Read the model definition and answer for the solid it produces. Units are mm, in the model's axes. Face numbers are marked on the shaded views. Give positions to 0.01 mm unless a question says otherwise; leave off trailing zeros. Order: outer loops, then holes, each group sorted by start corner. A loop starts at its lowest first (then second) coordinate and runs counter-clockwise, first axis right, second up. Notation, with made-up numbers: (4.5, 2) -> (27.5, 2) arc R22 ccw to (27.5, 10) -> close; hole circle Ø11 at (11.25, -38). An arc over 180 degrees is marked (long way). One line per question, with ' | ' between items. Start each with the question number.
```python
from build123d import *

# Parameters (mm, degrees)
PAD_DEPTH       = 5
SKETCH001_R     = 2.65
POCKET_DEPTH    = 5
SKETCH002_R     = 1.5
POCKET001_DEPTH = 5


with BuildPart() as part:
    # Sketch → Pad (new body)
    with BuildSketch(Plane.XY):
        Polygon((38.75, 34.75), (38.75, -34.75), (26.25, -34.75), (26.25, -45), (-38.75, -45), (-38.75, 45), (26.25, 45), (26.25, 34.75), align=None)
    extrude(amount=PAD_DEPTH)

    # Sketch001 (on Face10 of Pad) → Pocket (cut)
    with BuildSketch(Plane.XY.offset(5)):
        with Locations((31.25, 20)):
            Circle(SKETCH001_R)
        with Locations((31.25, -20)):
            Circle(SKETCH001_R)
    extrude(amount=-POCKET_DEPTH, mode=Mode.SUBTRACT)

    # Sketch002 (on Face5 of Pocket) → Pocket001 (cut)
    with BuildSketch(Plane.XY.offset(5)):
        with Locations((5.25, -16.5)):
            Circle(SKETCH002_R)
        with Locations((-16.75, -16.5)):
            Circle(SKETCH002_R)
        with Locations((-5.75, 15.5)):
            Circle(SKETCH002_R)
    extrude(amount=-POCKET001_DEPTH, mode=Mode.SUBTRACT)


solid = part.part
```
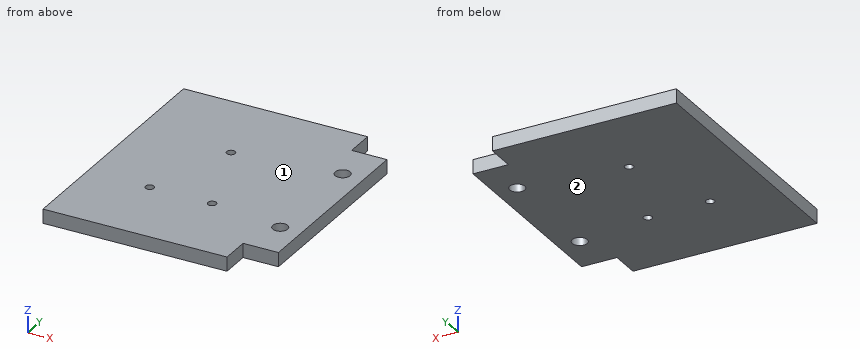
Q1. A cutting plane is placed at B-B, the plane y = -20. Determine the outline of the cut face in (x, z).
Q2. A cutting plane is placed at A-A, the plane x = 31.25. Determine the outline of the cut face in (y, z).
Q3. A cutting plane is placed at D-D, the plane x = 5.25. Determine the outline of the cut face in (y, z).
Q4. A cutting plane is placed at C-C, the plane z = 3.1. Determine the outline of the cut face in (x, y).
Q5. Given P1, Ø1.5, axis at x = 33.5, z = 1.5, coming from the +Y side; P2, Ø2.5, axis at x = 34, z = 1.5, coming from the -Y side; P3, Ø2.5, axis at y = 41.5, z = 2.5, coming from the +X side, each flat-ended and moving along its own axis, determine where each tip first touches the part or whether it passes through.
Q6. Determine the mould class of the marked faces 1 and 2 for opening direction Z: pulls with the +Z half, pulls with the -Z half, needs draft (parallel to the pull), parting line crosses it, or undercut.
Q7. Find the intervals of material crossed by line 1 (Y direction, x = 31.25, z = 3.6); line 2 (Y direction, x = -16.5, z = 2.6); line 3 (Y direction, x = -5.75, z = 1.65), in increasing order.
Geometry results:
1) outline: (-38.75, 0) -> (28.6, 0) -> (28.6, 5) -> (-38.75, 5) -> close; (33.9, 0) -> (38.75, 0) -> (38.75, 5) -> (33.9, 5) -> close
2) outline: (-34.75, 0) -> (-22.65, 0) -> (-22.65, 5) -> (-34.75, 5) -> close; (-17.35, 0) -> (17.35, 0) -> (17.35, 5) -> (-17.35, 5) -> close; (22.65, 0) -> (34.75, 0) -> (34.75, 5) -> (22.65, 5) -> close
3) outline: (-45, 0) -> (-18, 0) -> (-18, 5) -> (-45, 5) -> close; (-15, 0) -> (45, 0) -> (45, 5) -> (-15, 5) -> close
4) outline: (-38.75, -45) -> (26.25, -45) -> (26.25, -34.75) -> (38.75, -34.75) -> (38.75, 34.75) -> (26.25, 34.75) -> (26.25, 45) -> (-38.75, 45) -> close; hole circle Ø3 at (-16.75, -16.5); hole circle Ø3 at (-5.75, 15.5); hole circle Ø3 at (5.25, -16.5); hole circle Ø5.3 at (31.25, -20); hole circle Ø5.3 at (31.25, 20)
5) P1: y = 34.75 | P2: y = -34.75 | P3: x = 26.25
6) face 1: pulls with the +Z half | face 2: pulls with the -Z half
7) line 1: -34.75 to -22.65, -17.35 to 17.35, 22.65 to 34.75 | line 2: -45 to -17.98, -15.02 to 45 | line 3: -45 to 14, 17 to 45
